Geometry: final body of the model. Coordinates: model frame, mm. A direction names the side the tool comes from. Coordinates: 2 decimals unless noted, no trailing zeros. Order: outer loops, then holes, each group sorted by start corner. A loop starts at its lowest first (then second) coordinate and runs counter-clockwise, first axis right, second up. Notation, with made-up numbers: (73, 55.25) -> (125, 55.25) arc R27 cw to (125, 74.25) -> close; hole circle Ø10 at (72.25, 40.25). An arc over 180 degrees is marked (long way). Use one line per item in the form item = value.
```python
from build123d import *

# Parameters (mm, degrees)
BOSS_EXTRUDE1_DEPTH                          = 6.35
SKETCH3_R                                    = 3.5
CUT_EXTRUDE2_DEPTH                           = 139.002460895
SKETCH4_OUTSIDE_W                            = 133.666
SKETCH4_OUTSIDE_H                            = 145.76
CUT_EXTRUDE3_DEPTH                           = 139.002460895
FILLET1_R                                    = 10
CSK_FOR_5_16_FLAT_HEAD_MACHINE_SCREW_2_COUNT = 2
CSK_FOR_5_16_FLAT_HEAD_MACHINE_SCREW_2_PITCH = 38.1


with BuildPart() as part:
    # Sketch2 → Boss-Extrude1 (new body)
    with BuildSketch(Plane.XY):
        with BuildLine():
            Line((-10, -10), (-10, 103.338336241))
            Line((-10, 103.338336241), (62.358282022, 103.338336241))
            Line((62.358282022, 103.338336241), (91.244424357, 23.974312441))
            ThreePointArc((91.244424357, 23.974312441), (79.259842401, 5.488091998), (63.591736031, -10))
            Line((63.591736031, -10), (-10, -10))
        make_face()
    extrude(amount=BOSS_EXTRUDE1_DEPTH)

    # Sketch3 → Cut-Extrude2 (cut, through all)
    with BuildSketch(Plane.XY):
        with Locations((0, 70)):
            Circle(SKETCH3_R)
        with BuildLine():
            ThreePointArc((53.092633074, 89.324138098), (55.641638045, 79.811122038), (56.5, 70))
            ThreePointArc((56.5, 70), (60, 66.5), (63.5, 70))
            ThreePointArc((63.5, 70), (62.535292316, 81.026659282), (59.67048142, 91.718279101))
            ThreePointArc((59.67048142, 91.718279101), (55.184486746, 93.810132772), (53.092633074, 89.324138098))
        make_face()
        with BuildLine():
            ThreePointArc((77.273680119, 26.460819381), (68.539219913, 13.703843633), (57.722230193, 2.657398108))
            ThreePointArc((57.722230193, 2.657398108), (57.342601892, -2.277769807), (62.277769807, -2.657398108))
            ThreePointArc((62.277769807, -2.657398108), (73.948455322, 9.260852265), (83.372254441, 23.024630908))
            ThreePointArc((83.372254441, 23.024630908), (82.041061517, 27.792012306), (77.273680119, 26.460819381))
        make_face()
        with BuildLine():
            ThreePointArc((22.744339531, 7.510440718), (11.547603815, 4.510284425), (0, 3.5))
            ThreePointArc((0, 3.5), (-3.5, 0), (0, -3.5))
            ThreePointArc((0, -3.5), (12.763141059, -2.383369846), (25.138480534, 0.932592372))
            ThreePointArc((25.138480534, 0.932592372), (27.230334206, 5.418587047), (22.744339531, 7.510440718))
        make_face()
    extrude(amount=CUT_EXTRUDE2_DEPTH, mode=Mode.SUBTRACT)

    # Sketch4 outside → Cut-Extrude3 (cut, through all)
    with BuildSketch(Plane.XY):
        with Locations((40.622, 46.669)):
            Rectangle(SKETCH4_OUTSIDE_W, SKETCH4_OUTSIDE_H)
        with BuildLine():
            Line((65.893010444, 46.375623296), (52.822036509, 9.918118713))
            ThreePointArc((52.822036509, 9.918118713), (28.226313052, -4.855028231), (0, -10))
            Line((0, -10), (-10, -10))
            Line((-10, -10), (-10, 74.111503744))
            Line((-10, 74.111503744), (6.084489401, 97.400118036))
            Line((6.084489401, 97.400118036), (62.358282022, 103.338336241))
            Line((62.358282022, 103.338336241), (65.778483455, 93.941410033))
            ThreePointArc((65.778483455, 93.941410033), (69.999797095, 70.168542697), (65.893010444, 46.375623296))
        make_face(mode=Mode.SUBTRACT)
    extrude(amount=CUT_EXTRUDE3_DEPTH, mode=Mode.SUBTRACT)

    # Fillet1
    fillet1_edges = [part.edges().sort_by_distance(p)[0] for p in [
        (52.822036509, 9.918118713, 3.175),
        (-10, -10, 3.175),
        (-10, 74.111503744, 3.175),
        (62.358282022, 103.338336241, 3.175),
        (6.084489401, 97.400118036, 3.175),
    ]]
    fillet(fillet1_edges, radius=FILLET1_R - 0.0001)  # a hair under: the kernel refuses the full size

    # Sketch9 → CSK for 5_16 Flat Head Machine Screw _10 (revolve, cut)
    with BuildSketch(Plane(origin=(28.384975395, 71.315714753, 0), x_dir=(0, 1, 0), z_dir=(1, 0, 0))):
        Polygon((0, 0), (0, 6.35), (4.2164, 6.35), (4.2164, 3.228939291), (8.0645, 0), align=None)
    csk_for_5_16_flat_head_machine_screw_10 = revolve(axis=Axis((28.384975395, 71.315714753, -6.35), (0, 0, 1)), mode=Mode.SUBTRACT)

    # CSK for 5_16 Flat Head Machine Screw 2: CSK for 5_16 Flat Head Machine Screw _10 ×2
    with Locations(*[(0, -i * CSK_FOR_5_16_FLAT_HEAD_MACHINE_SCREW_2_PITCH, 0) for i in range(1, CSK_FOR_5_16_FLAT_HEAD_MACHINE_SCREW_2_COUNT)]):
        add(csk_for_5_16_flat_head_machine_screw_10, mode=Mode.SUBTRACT)


solid = part.part
```
1) Section A-A, the plane y = 87.5. Output: boundary loops of the cut face in (x, z).
Results found:
outline = (-0.75, 0) -> (53.72, 0) -> (53.72, 6.35) -> (-0.75, 6.35) -> close; (61.04, 0) -> (67.78, 0) -> (67.78, 6.35) -> (61.04, 6.35) -> close
2) Access query for faces 4 (the conical face through (32.339, 35.272, 3.027)), 5 (the cylindrical face through (59.9, 66.5, 3.1)). Directions: +Z, -Z, +X, -X, +Y, -Y. A direction counts if a zero-diameter tool reaches every point of the face in a straight line with its end or side. Return the directions, or none.
Results found:
face_4 = -Z
face_5 = +Z, -Z
3) Section C-C, the plane z = 1.5. Give the number of separate pieces and of enclosed holes in the cut face, and give its area (3 significant figures).
Results found:
separate_pieces = 1
enclosed_holes = 5
area = 6,720 mm2
4) Material intervals for probe 1 along Y at (x, z) = (32, 4.5); probe 2 along Y at (x, z) = (26, 5.5); probe 3 along Y at (x, z) = (13, 2), sorted ascending. Write a range as from..to.
Results found:
probe_1 = -3.32..31.05, 35.39..69.15, 73.49..100.13
probe_2 = -5.66..1.39, 7.05..29.74, 36.69..67.84, 74.79..99.5
probe_3 = -8.94..-2.34, 4.78..98.13
5) Contact query for flat-ended pins moving along their axis: P1, Ø4, axis at x = 0, y = 70, coming from the -Z side; P2, Ø1, axis at y = 78, z = 1, coming from the +X side; P3, Ø3, axis at x = 52, z = 2.5, coming from the +Y side; P4, Ø11, axis at x = 28.38, y = 33.22, coming from the -Z side. Output: stop coordinate, or through.
Results found:
P1 = through
P2 = 69.6
P3 = 102.4
P4 = 2.15
6) Pull-direction query (X, two-part tool) for faces 1 (the cylindrical face through (62.562, 80.874, 3.131)), 2 (the cylindrical face through (70, 70.5, 3.1)), 3 (the cylindrical face through (-9.56, 73.93, 3.22)); classes: released by +X, released by -X, zero draft, split by the parting line, or undercut.
Results found:
face_1 = undercut
face_2 = released by +X
face_3 = released by -X
7) Section B-B, the plane x = 62. Output: boundary loops of the cut face in (y, z), and give its area (3 significant figures).
Results found:
outline = (35.52, 0) -> (67.13, 0) -> (67.13, 6.35) -> (35.52, 6.35) -> close; (83.72, 0) -> (100.29, 0) -> (100.29, 6.35) -> (83.72, 6.35) -> close
area = 306 mm2
